```python
from build123d import *

# Parameters (mm, degrees)
BOSS_EXTRUDE1_DEPTH = 730.25
SKETCH2_R           = 12.7
CUT_EXTRUDE1_DEPTH  = 3.175
LPATTERN1_COUNT     = 3
LPATTERN1_PITCH     = 420.6875


with BuildPart() as part:
    # Sketch1 → Boss-Extrude1 (new body, symmetric)
    with BuildSketch(Plane(origin=(0, 0, 0), x_dir=(0, 0, -1), z_dir=(1, 0, 0))):
        with BuildLine():
            Line((33.3248, 25.4), (-33.3248, 25.4))
            ThreePointArc((-33.3248, 25.4), (-36.701376302, 24.001376302), (-38.1, 20.6248))
            Line((-38.1, 20.6248), (-38.1, 4.7752))
            ThreePointArc((-38.1, 4.7752), (-36.701376302, 1.398623698), (-33.3248, 0))
            Line((-33.3248, 0), (33.3248, 0))
            ThreePointArc((33.3248, 0), (36.701376302, 1.398623698), (38.1, 4.7752))
            Line((38.1, 4.7752), (38.1, 20.6248))
            ThreePointArc((38.1, 20.6248), (36.701376302, 24.001376302), (33.3248, 25.4))
        make_face()
        with BuildLine():
            Line((33.3248, 22.225), (-33.3248, 22.225))
            ThreePointArc((-33.3248, 22.225), (-34.456312271, 21.756312271), (-34.925, 20.6248))
            Line((-34.925, 20.6248), (-34.925, 4.7752))
            ThreePointArc((-34.925, 4.7752), (-34.456312271, 3.643687729), (-33.3248, 3.175))
            Line((-33.3248, 3.175), (33.3248, 3.175))
            ThreePointArc((33.3248, 3.175), (34.456312271, 3.643687729), (34.925, 4.7752))
            Line((34.925, 4.7752), (34.925, 20.6248))
            ThreePointArc((34.925, 20.6248), (34.456312271, 21.756312271), (33.3248, 22.225))
        make_face(mode=Mode.SUBTRACT)
    extrude(amount=BOSS_EXTRUDE1_DEPTH, both=True)

    # Sketch2 → Cut-Extrude1 (cut)
    with BuildSketch(Plane(origin=(0, 25.4, 0), x_dir=(1, 0, 0), z_dir=(0, 1, 0))):
        with Locations((-420.6875, 0)):
            Circle(SKETCH2_R)
    cut_extrude1 = extrude(amount=-CUT_EXTRUDE1_DEPTH, mode=Mode.SUBTRACT)

    # LPattern1: Cut-Extrude1 ×3
    with Locations(*[(i * LPATTERN1_PITCH, 0, 0) for i in range(1, LPATTERN1_COUNT)]):
        add(cut_extrude1, mode=Mode.SUBTRACT)


solid = part.part
```
The model under review builds one solid part; all positions refer to its coordinate system, in mm. A direction names the side the tool comes from. Give positions to 0.01 mm unless a question says otherwise; leave off trailing zeros. Write each loop counter-clockwise with the first axis right and the second up, starting at its lowest first coordinate (ties: lowest second). Pieces come first, ordered by that corner, then holes. Notation, with made-up numbers: M 87,35.5 L 100,35.5 A24 ccw 100,60.5 Z; hole C -33.5,-3.75 d11. An arc over 180 degrees is marked long. Write item = value, one per line. Start each with the question number.
Q1. We need section A-A (z = 0). Give the number of separate pieces and of enclosed holes in the cut face, plus the area to 3 significant figures.
Q2. Mouldability with a two-part tool opening along X and no side actions: class faces 4 (the face through (10.2, 25.4, -7.9)), 5 (the face through (730.25, 23, 3)), 6 (the face through (-730.25, 23, 3)), 7 (the face through (-408.574, 23.835, -3.815)) as released by +X, released by -X, zero draft, split by the parting line, or undercut.
Q3. Machinability: for faces 1 (the face through (10.2, 22.225, -7.9)), 2 (the face through (10, 0, 0)), 3 (the face through (432.801, 23.835, -3.815)), which of the approach directions +Z, -Z, +X, -X, +Y, -Y give a long, thin tool a straight path to every point of the face, cutting with its end or side? Answer none if there is none.
Q4. We need section B-B (y = 11.5). State the section outline as (x, z) points (3 decimals), plus the area to 3 significant figures.
Q5. We need section C-C (x = -284.5). State the section outline as (y, z) points (3 decimals), plus the area to 3 significant figures.
Q6. For line 1 (X direction, y = 24.45, z = 0); line 2 (Z direction, x = -191.5, y = 7.5) (3 decimals); line 3 (Y direction, x = 326.5, z = -16) (3 decimals), list the stretches that pass through material, from the lowest coordinate up.
Q7. We need section D-D (x = 0). State the section outline as (y, z) points (3 decimals).
Result set:
q1.separate_pieces = 5
q1.enclosed_holes = 0
q1.area = 9,030 mm2
q2.face_4 = zero draft
q2.face_5 = released by +X
q2.face_6 = released by -X
q2.face_7 = undercut
q3.face_1 = +X, -X
q3.face_2 = +Z, -Z, +X, -X, -Y
q3.face_3 = +Y
q4.outline = M -730.25,-38.1 L 730.25,-38.1 L 730.25,-34.925 L -730.25,-34.925 Z; M -730.25,34.925 L 730.25,34.925 L 730.25,38.1 L -730.25,38.1 Z
q4.area = 9,270 mm2
q5.outline = M 0,-33.325 A4.775 ccw 4.775,-38.1 L 20.625,-38.1 A4.775 ccw 25.4,-33.325 L 25.4,33.325 A4.775 ccw 20.625,38.1 L 4.775,38.1 A4.775 ccw 0,33.325 Z; hole M 3.175,-33.325 A1.6 ccw 4.775,-34.925 L 20.625,-34.925 A1.6 ccw 22.225,-33.325 L 22.225,33.325 A1.6 ccw 20.625,34.925 L 4.775,34.925 A1.6 ccw 3.175,33.325 Z
q5.area = 587 mm2
q6.line_1 = -730.25 to -433.39, -407.99 to -12.7, 12.7 to 407.99, 433.39 to 730.25
q6.line_2 = -38.1 to -34.925, 34.925 to 38.1
q6.line_3 = 0 to 3.175, 22.225 to 25.4
q7.outline = M 0,-33.325 A4.775 ccw 4.775,-38.1 L 20.625,-38.1 A4.775 ccw 25.4,-33.325 L 25.4,-12.7 L 22.225,-12.7 L 22.225,-33.325 A1.6 cw 20.625,-34.925 L 4.775,-34.925 A1.6 cw 3.175,-33.325 L 3.175,33.325 A1.6 cw 4.775,34.925 L 20.625,34.925 A1.6 cw 22.225,33.325 L 22.225,12.7 L 25.4,12.7 L 25.4,33.325 A4.775 ccw 20.625,38.1 L 4.775,38.1 A4.775 ccw 0,33.325 Z
